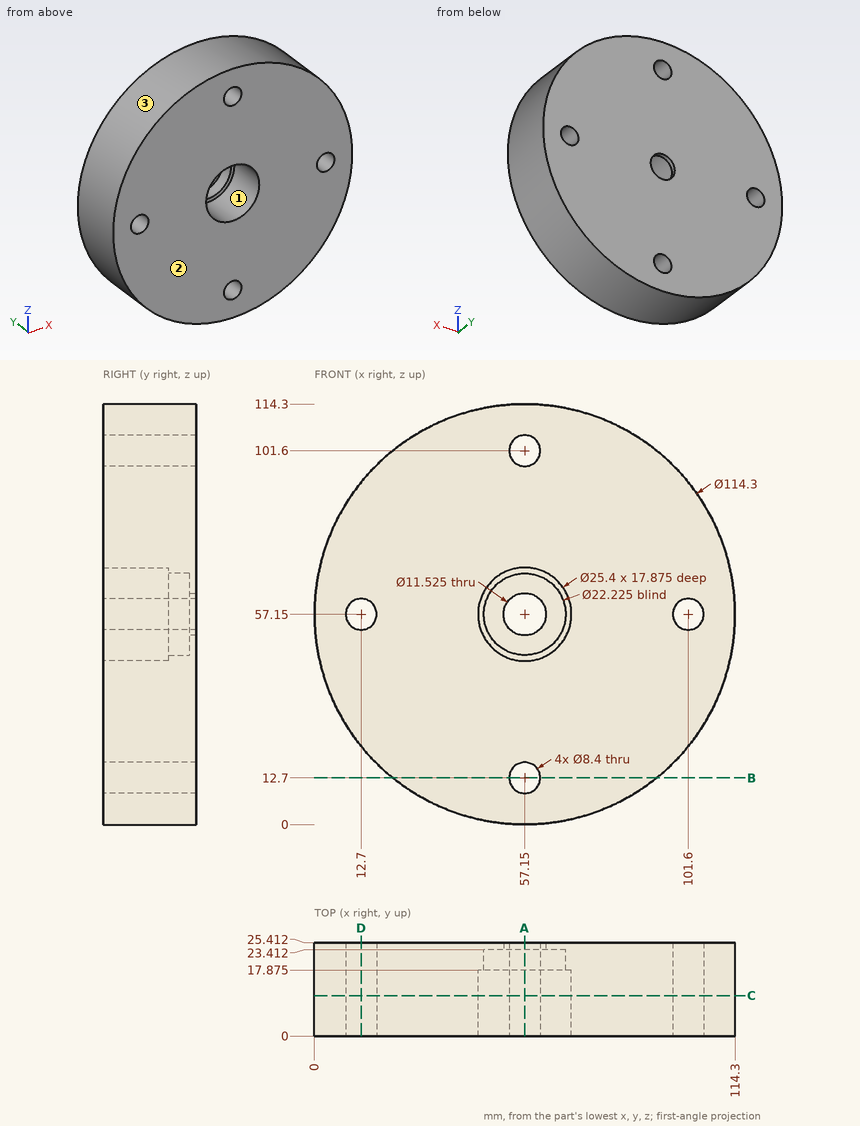
For this review, use the dimensioned drawing (mm, ordinates from the lowest corner) and the shaded views. Round coordinates to 2 decimals unless told otherwise and drop trailing zeros. Write each loop counter-clockwise with the first axis right and the second up, starting at its lowest first coordinate (ties: lowest second). Pieces come first, ordered by that corner, then holes. Notation, with made-up numbers: M 30.25,81.5 L 45.25,81.5 A21 ccw 45.25,119.5 Z; hole C 1,10 d9. An arc over 180 degrees is marked long. Write item = value, one per line. Start each with the question number.
(1) We need section C-C (y = 11). Give the boundary of the cut face in (x, z), then the cut area to 3 significant figures.
(2) We need section B-B (z = 12.7). Give the boundary of the cut face in (x, y).
(3) We need section A-A (x = 57.15). Give the number of separate pieces and of enclosed holes in the cut face, then the cut area to 3 significant figures.
(4) The part is to be moulded in two halves that separate along Z. For the marked faces 1, 2 and 3, say which applies: +Z half, -Z half, draft (parallel to the pull), parting line (faces both ways), or undercut.
(5) We need section D-D (x = 12.7). Give the boundary of the cut face in (y, z).
(6) For line 1 along X through (y, z) = (5.5, 57.15); line 2 along X through (y, z) = (19.1, 57.15); line 3 along X through (y, z) = (5.75, 12.7), list the stretches that pass through material, from the lowest coordinate up.
(7) Clearance check with flat-ended pins moving along their axes: pin 1 Ø3 at (x, y) = (79, 11.5) entering from +Z; pin 2 Ø4 at (y, z) = (5, 61.5) entering from -X; pin 3 Ø10 at (y, z) = (21.5, 76.5) entering from -X; pin 4 Ø13.5 at (x, z) = (57.15, 101.6) entering from -Y. State where each tip first meets the part, or that it passes through.
Results found:
q1.outline = C 57.15,57.15 d114.3; hole C 12.7,57.15 d8.4; hole C 57.15,57.15 d25.4; hole C 57.15,12.7 d8.4; hole C 57.15,101.6 d8.4; hole C 101.6,57.15 d8.4
q1.area = 9,530 mm²
q2.outline = M 21.23,0 L 52.95,0 L 52.95,25.41 L 21.23,25.41 Z; M 61.35,0 L 93.07,0 L 93.07,25.41 L 61.35,25.41 Z
q3.separate_pieces = 4
q3.enclosed_holes = 0
q3.area = 1,880 mm²
q4.face_1 = undercut
q4.face_2 = draft
q4.face_3 = parting line
q5.outline = M 0,21.23 L 25.41,21.23 L 25.41,52.95 L 0,52.95 Z; M 0,61.35 L 25.41,61.35 L 25.41,93.07 L 0,93.07 Z
q6.line_1 = 0 to 8.5, 16.9 to 44.45, 69.85 to 97.4, 105.8 to 114.3
q6.line_2 = 0 to 8.5, 16.9 to 46.04, 68.26 to 97.4, 105.8 to 114.3
q6.line_3 = 21.23 to 52.95, 61.35 to 93.07
q7.pin_1 = 110.55
q7.pin_2 = 0.05
q7.pin_3 = 1.83
q7.pin_4 = 0
